Source: CAD feature listing. Evaluate the final solid. Frame: model axes, mm. Face numbers are marked on the shaded views. Coordinates: 2 decimals unless noted, no trailing zeros. Write each loop counter-clockwise with the first axis right and the second up, starting at its lowest first coordinate (ties: lowest second). Pieces come first, ordered by that corner, then holes. Notation, with made-up numbers: (72, 51) - (92, 51) arc R17 cw to (92, 82) - close; hole circle Ø1 at (81.5, 14). An arc over 180 degrees is marked (long way). One line per item, written item: value.
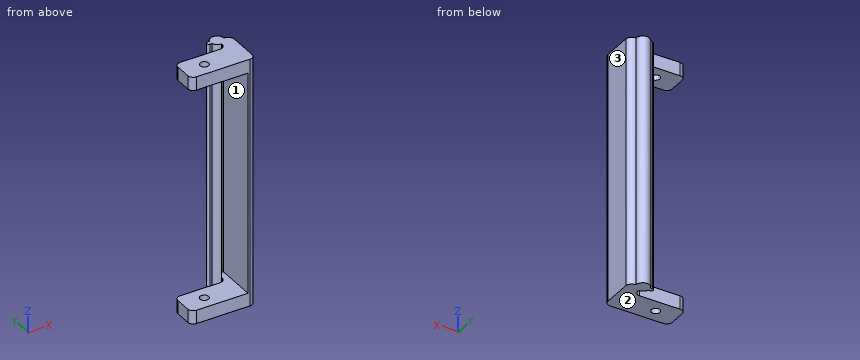
from build123d import *

# Parameters (mm, degrees)
SKETCH1_R           = 1.6
BOSS_EXTRUDE1_DEPTH = 93
SKETCH3_W           = 21.267787972
SKETCH3_H           = 83
CUT_EXTRUDE2_DEPTH  = 90
BOSS_EXTRUDE4_REACH = 99.216


with BuildPart() as part:
    # Sketch1 → Boss-Extrude1 (new body)
    with BuildSketch(Plane.XY):
        with BuildLine():
            Line((17.033489737, 10), (2, 10))
            ThreePointArc((2, 10), (0.585786438, 9.414213562), (0, 8))
            Line((0, 8), (0, 2))
            ThreePointArc((0, 2), (0.585786438, 0.585786438), (2, 0))
            Line((2, 0), (20.255670014, 0))
            Line((20.255670014, 0), (22, 0))
            ThreePointArc((22, 0), (23.414213562, 0.585786438), (24, 2))
            Line((24, 2), (24, 10))
            Line((24, 10), (24, 13))
            ThreePointArc((24, 13), (21.016744869, 14.983255131), (19.033489737, 12))
            ThreePointArc((19.033489737, 12), (18.447703299, 10.585786438), (17.033489737, 10))
        make_face()
        with Locations(Location((8.031280577, 5, 0), (0, 0, 180))):
            Circle(SKETCH1_R, mode=Mode.SUBTRACT)
    extrude(amount=BOSS_EXTRUDE1_DEPTH)

    # Sketch3 → Cut-Extrude2 (cut)
    with BuildSketch(Plane(origin=(0, 15, 0), x_dir=(1, 0, 0), z_dir=(0, 1, 0))):
        with Locations((10.633893986, -46.5)):
            Rectangle(SKETCH3_W, SKETCH3_H)
    extrude(amount=-CUT_EXTRUDE2_DEPTH, mode=Mode.SUBTRACT)

    # Boss-Extrude4: up to this face of the body (flat: up to its plane)
    boss_extrude4_end = Plane(part.part.faces().sort_by_distance((13.034633822, 5.682959989, 0))[0])
    # Sketch4 → Boss-Extrude4 (add, up to the picked face)
    with BuildSketch(Plane.XY.offset(93), mode=Mode.PRIVATE) as boss_extrude4_sk1:
        with BuildLine():
            ThreePointArc((21.516744869, 15.033092191), (19.36575731, 17.537199237), (16.565837736, 15.78855692))
            Line((16.565837736, 15.78855692), (15.846137498, 15.78855692))
            ThreePointArc((15.846137498, 15.78855692), (15.090672769, 15.033092191), (15.846137498, 14.277627462))
            Line((15.846137498, 14.277627462), (16.565837736, 14.277627462))
            ThreePointArc((16.565837736, 14.277627462), (17.483170381, 12.992232341), (18.983652678, 12.5))
            ThreePointArc((18.983652678, 12.5), (19.725578203, 14.291166666), (21.516744869, 15.033092191))
        make_face()
    boss_extrude4_tool1 = split(extrude(boss_extrude4_sk1.sketch, amount=-BOSS_EXTRUDE4_REACH, mode=Mode.PRIVATE), bisect_by=boss_extrude4_end, keep=Keep.BOTH, mode=Mode.PRIVATE)
    add(boss_extrude4_tool1.solids().sort_by(Axis((18.413371, 15.285709, 93), (0, 0, -1)))[0])


solid = part.part
1) Section query B-B on x = 3.25. Output: boundary loops of the cut face in (y, z).
Values found:
outline: (0, 0) - (10, 0) - (10, 5) - (0, 5) - close; (0, 88) - (10, 88) - (10, 93) - (0, 93) - close
2) Material intervals for line 1 (Z direction, x = 19.75, y = 4); line 2 (X direction, y = 5, z = 3.6); line 3 (X direction, y = 4, z = 70.5), sorted ascending.
Values found:
line 1: 0 to 5, 88 to 93
line 2: 0 to 6.43, 9.63 to 24
line 3: 21.27 to 24
3) Section query A-A on y = 5. Output: boundary loops of the cut face in (x, z), then the cut area to 3 significant figures.
Values found:
outline: (0, 0) - (6.43, 0) - (6.43, 5) - (0, 5) - close; (0, 88) - (6.43, 88) - (6.43, 93) - (0, 93) - close; (9.63, 0) - (24, 0) - (24, 93) - (9.63, 93) - (9.63, 88) - (21.27, 88) - (21.27, 5) - (9.63, 5) - close
area: 435 mm2
4) Section query C-C on z = 36. Output: boundary loops of the cut face in (x, y), then the cut area to 3 significant figures.
Values found:
outline: (15.85, 14.28) - (16.57, 14.28) arc R2.53 ccw to (18.98, 12.5) arc R2.53 cw to (21.11, 15) - (21.27, 15) - (21.27, 0) - (22, 0) arc R2 ccw to (24, 2) - (24, 13) arc R2.53 ccw to (21.52, 15.03) arc R2.53 ccw to (16.57, 15.79) - (15.85, 15.79) arc R0.76 ccw to start
area: 57.3 mm2
5) Draft query along Z for the marked faces 1, 2 and 3. Return one class per face: released by +Z, released by -Z, zero draft, split by the parting line, or undercut.
Values found:
face 1: undercut
face 2: released by -Z
face 3: zero draft
6) Contact query for flat-ended pins moving along their axis: P1, Ø3, axis at y = 15, z = 16, coming from the -X side; P2, Ø0.6, axis at x = 16, z = 64.5, coming from the -Y side; P3, Ø3, axis at x = 17, z = 13, coming from the -Y side; P4, Ø3, axis at x = 20, y = 4.5, coming from the -Z side. Output: stop coordinate, or through.
Values found:
P1: x = 15.09
P2: y = 14.28
P3: y = 12.55
P4: z = 0
